```python
from build123d import *

# Parameters (mm, degrees)
BASE_PROFILE_SKETCH_W          = 12.001239904
BASE_PROFILE_SKETCH_H          = 15.00124
BASE_PROFILE_EXTRUDE_DEPTH     = 3
BACK_PROFILE_SKETCH_W          = 12.001239904
BACK_PROFILE_SKETCH_H          = 3
BACK_PROFILE_EXTRUDE_DEPTH     = 15
SIDE_PROFILE_EXTRUDE_DEPTH     = 3
BOTTOM_MOUNTING_HOLE_CUT_REACH = 5
BOTTOM_MOUNTING_HOLE_SKETCH_R  = 1.575
BACK_MOUNTING_HOLE_CUT_REACH   = 5
BACK_MOUNTING_HOLE_SKETCH_R    = 1.575


with BuildPart() as part:
    # Base Profile Sketch → Base Profile Extrude (new body)
    with BuildSketch(Plane.XY):
        Rectangle(BASE_PROFILE_SKETCH_W, BASE_PROFILE_SKETCH_H)
    extrude(amount=BASE_PROFILE_EXTRUDE_DEPTH)

    # Back Profile Sketch → Back Profile Extrude (add)
    with BuildSketch(Plane.XY.offset(3)):
        with Locations((0, -6.00062)):
            Rectangle(BACK_PROFILE_SKETCH_W, BACK_PROFILE_SKETCH_H)
    extrude(amount=BACK_PROFILE_EXTRUDE_DEPTH)

    # Side Profile Sketch → Side Profile Extrude (add)
    with BuildSketch(Plane(origin=(6.000619952, 0, 0), x_dir=(0, 0, -1), z_dir=(1, 0, 0))):
        Polygon((0, -7.50062), (0, 7.50062), (-3, 7.50062), (-18, -4.50062), (-18, -7.50062), align=None)
    extrude(amount=SIDE_PROFILE_EXTRUDE_DEPTH)

    # Bottom Mounting Hole Sketch → Bottom Mounting Hole Cut (cut, up to next)
    with BuildSketch(Plane.XY.offset(3), mode=Mode.PRIVATE) as bottom_mounting_hole_cut_sk1:
        with Locations((1.5, 1.5)):
            Circle(BOTTOM_MOUNTING_HOLE_SKETCH_R)
    bottom_mounting_hole_cut_tool1 = extrude(bottom_mounting_hole_cut_sk1.sketch, amount=-BOTTOM_MOUNTING_HOLE_CUT_REACH, mode=Mode.PRIVATE) & part.part
    add(bottom_mounting_hole_cut_tool1.solids().sort_by_distance((1.5, 1.5, 3))[0], mode=Mode.SUBTRACT)

    # Back Mounting Hole Sketch → Back Mounting Hole Cut (cut, up to next)
    with BuildSketch(Plane(origin=(0, -4.50062, 0), x_dir=(1, 0, 0), z_dir=(0, 1, 0)), mode=Mode.PRIVATE) as back_mounting_hole_cut_sk1:
        with Locations((1.5, -10.5)):
            Circle(BACK_MOUNTING_HOLE_SKETCH_R)
    back_mounting_hole_cut_tool1 = extrude(back_mounting_hole_cut_sk1.sketch, amount=-BACK_MOUNTING_HOLE_CUT_REACH, mode=Mode.PRIVATE) & part.part
    add(back_mounting_hole_cut_tool1.solids().sort_by_distance((1.5, -4.50062, 10.5))[0], mode=Mode.SUBTRACT)


solid = part.part
```
The listing builds one solid part. Answer for the finished solid, in the listing's coordinates (mm). A direction names the side the tool comes from. Give positions to 0.01 mm unless a question says otherwise; leave off trailing zeros. Order: outer loops, then holes, each group sorted by start corner. A loop starts at its lowest first (then second) coordinate and runs counter-clockwise, first axis right, second up. Notation, with made-up numbers: (9.5, 9) - (45.5, 9) arc R5 cw to (45.5, 14) - close; hole circle Ø1 at (5.5, 37). An arc over 180 degrees is marked (long way). Answer in a Markdown table with one row per item. Add a question column.
Q1. For a pull along Y with two mould halves and no side action, classify faces 3 (the cylindrical face through (3.002, 1.973, 1.521)), 4 (the flat face through (-6.001, -5, 5)), 5 (the flat face through (1, 7.501, 1)) as released by +Y, released by -Y, zero draft, split by the parting line, or undercut.
Q2. Given P1, Ø5, axis at x = 1.5, y = 1.5, coming from the +Z side; P2, Ø3, axis at x = 1.5, z = 10.5, coming from the -Y side; P3, Ø4, axis at x = 7, y = -0.5, coming from the +Z side, each flat-ended and moving along its own axis, determine where each tip first touches the part or whether it passes through.
Q3. Find the intervals of material crossed by line 1 along Y through (x, z) = (1.5, 0.75) (3 decimals); line 2 along Y through (x, z) = (-0.25, 3.5); line 3 along X through (y, z) = (-3.25, 14), in increasing order. Write a range as [from, to].
Q4. The part is cut by section D-D (z = 2). Determine the outline of the cut face in (x, y) (3 decimals), then the cut area to 3 significant figures.
Q5. The part is cut by section A-A (z = 10.5). Determine the outline of the cut face in (x, y) (3 decimals), then the cut area to 3 significant figures.
Q6. The part is cut by section B-B (x = 1.5). Determine the outline of the cut face in (y, z) (3 decimals), then the cut area to 3 significant figures.
Q7. The part is cut by section C-C (y = 1.5). Determine the outline of the cut face in (x, z) (3 decimals).
Q8. Which of the six approach directions +Z, -Z, +X, -X, +Y, -Y give full straight-line access (tool end or side, diameter ignored) to faces 1 (the flat face through (0, -7.501, 9)), 2 (the flat face through (-1, -4.501, 10))?
Determined:
| question | item | result |
|---|---|---|
| 1 | face 3 | undercut |
| 1 | face 4 | zero draft |
| 1 | face 5 | released by +Y |
| 2 | P1 | stops at z = 3 |
| 2 | P2 | passes through |
| 2 | P3 | stops at z = 15.5 |
| 3 | line 1 | y = [-7.501, -0.075], [3.075, 7.501] |
| 3 | line 2 | y = [-7.5, -4.5] |
| 3 | line 3 | x = [6, 9] |
| 4 | outline | (-6.001, -7.501) - (9.001, -7.501) - (9.001, 7.501) - (-6.001, 7.501) - close; hole circle Ø3.15 at (1.5, 1.5) |
| 4 | area | 217 mm² |
| 5 | outline | (-6.001, -7.501) - (-0.075, -7.501) - (-0.075, -4.501) - (-6.001, -4.501) - close; (3.075, -7.501) - (9.001, -7.501) - (9.001, 1.5) - (6.001, 1.5) - (6.001, -4.501) - (3.075, -4.501) - close |
| 5 | area | 53.6 mm² |
| 6 | outline | (-7.501, 0) - (-0.075, 0) - (-0.075, 3) - (-4.501, 3) - (-4.501, 8.925) - (-7.501, 8.925) - close; (-7.501, 12.075) - (-4.501, 12.075) - (-4.501, 18) - (-7.501, 18) - close; (3.075, 0) - (7.501, 0) - (7.501, 3) - (3.075, 3) - close |
| 6 | area | 71.1 mm² |
| 7 | outline | (-6.001, 0) - (-0.075, 0) - (-0.075, 3) - (-6.001, 3) - close; (3.075, 0) - (9.001, 0) - (9.001, 10.5) - (6.001, 10.5) - (6.001, 3) - (3.075, 3) - close |
| 8 | face 1 | +Z, -Z, +X, -X, -Y |
| 8 | face 2 | +Z, -X, +Y |
